Can you work these out from the model? Positions are in its coordinate system, mm. A direction names the side the tool comes from. Coordinates: 2 decimals unless noted, no trailing zeros. Order: outer loops, then holes, each group sorted by start corner. A loop starts at its lowest first (then second) coordinate and runs counter-clockwise, first axis right, second up.
```python
from build123d import *

# Parameters (mm, degrees)
SKETCH_1_W          = 50
SKETCH_1_H          = 50
SKETCH_1_R          = 1.6
EXTRUDE_1_DEPTH     = 20
SKETCH_2_W          = 45
SKETCH_2_H          = 26
CUT_EXTRUDE_1_DEPTH = 16.5
SKETCH_4_R          = 4.6
CUT_EXTRUDE_2_DEPTH = 15
SKETCH_5_R          = 5.15
CUT_EXTRUDE_3_DEPTH = 0.6
CHAMFER_1_SIZE      = 5
SKETCH_6_R          = 3.75
CUT_EXTRUDE_4_DEPTH = 3.3
SKETCH_7_R          = 15
CUT_EXTRUDE_5_DEPTH = 16.5
FILLET_1_R          = 10


with BuildPart() as part:
    # 草图1 → 凸台-拉伸1 (new body)
    with BuildSketch(Plane(origin=(0, 0, 0), x_dir=(1, 0, 0), z_dir=(0, 1, 0))):
        with Locations((25, 25)):
            Rectangle(SKETCH_1_W, SKETCH_1_H)
        with Locations((13.65, 40.5)):
            Circle(SKETCH_1_R, mode=Mode.SUBTRACT)
        with Locations((44.65, 40.5)):
            Circle(SKETCH_1_R, mode=Mode.SUBTRACT)
        with Locations((44.65, 9.5)):
            Circle(SKETCH_1_R, mode=Mode.SUBTRACT)
        with Locations((13.65, 9.5)):
            Circle(SKETCH_1_R, mode=Mode.SUBTRACT)
    extrude(amount=EXTRUDE_1_DEPTH)

    # 草图2 → 切除-拉伸1 (cut)
    with BuildSketch(Plane.XZ):
        with Locations((27.5, -25)):
            Rectangle(SKETCH_2_W, SKETCH_2_H)
    extrude(amount=-CUT_EXTRUDE_1_DEPTH, mode=Mode.SUBTRACT)

    # 草图4 → 切除-拉伸2 (cut)
    with BuildSketch(Plane(origin=(0, 20, 0), x_dir=(1, 0, 0), z_dir=(0, 1, 0))):
        with Locations((29.15, 25)):
            Circle(SKETCH_4_R)
    extrude(amount=-CUT_EXTRUDE_2_DEPTH, mode=Mode.SUBTRACT)

    # 草图5 → 切除-拉伸3 (cut)
    with BuildSketch(Plane.XZ.offset(-16.5)):
        with Locations((29.15, -25)):
            Circle(SKETCH_5_R)
    extrude(amount=-CUT_EXTRUDE_3_DEPTH, mode=Mode.SUBTRACT)

    # 倒角1
    chamfer_1_edges = [part.edges().sort_by_distance(p)[0] for p in [
        (25, 20, -50),
        (50, 8.25, -12),
        (50, 8.25, -38),
        (0, 20, -25),
        (0, 10, -50),
        (50, 10, -50),
        (50, 10, 0),
        (0, 10, 0),
        (25, 20, 0),
    ]]
    chamfer(chamfer_1_edges, length=CHAMFER_1_SIZE)

    # 草图6 → 切除-拉伸4 (cut)
    with BuildSketch(Plane(origin=(0, 20, 0), x_dir=(1, 0, 0), z_dir=(0, 1, 0))):
        with Locations((13.65, 40.5)):
            Circle(SKETCH_6_R)
        with Locations((44.65, 40.5)):
            Circle(SKETCH_6_R)
        with Locations((44.65, 9.5)):
            Circle(SKETCH_6_R)
        with Locations((13.65, 9.5)):
            Circle(SKETCH_6_R)
    extrude(amount=-CUT_EXTRUDE_4_DEPTH, mode=Mode.SUBTRACT)

    # 草图7 → 切除-拉伸5 (cut)
    with BuildSketch(Plane.XZ):
        with Locations((29.15, -25)):
            Circle(SKETCH_7_R)
    extrude(amount=-CUT_EXTRUDE_5_DEPTH, mode=Mode.SUBTRACT)

    # 圆角1
    fillet_1_edges = [part.edges().sort_by_distance(p)[0] for p in [
        (21.666685226, 8.25, -12),
        (36.633314774, 8.25, -12),
        (36.633314774, 8.25, -38),
        (21.666685226, 8.25, -38),
    ]]
    fillet(fillet_1_edges, radius=FILLET_1_R)


solid = part.part
```
1. Please list where these lines run through material, in increasing order: probe 1 along Z at (x, y) = (13.65, 8); probe 2 along X at (y, z) = (18.9, -40.5); probe 3 along Z at (x, y) = (13.65, 19.35).
Completed:
probe 1: z = -50 to -42.1, -38.9 to -38, -12 to -11.1, -7.9 to 0
probe 2: x = 3.9 to 9.9, 17.4 to 40.9, 48.4 to 50
probe 3: z = -45.65 to -44.25, -36.75 to -13.25, -5.75 to -4.35
2. On a 3-axis mill with a long thin cutter (end or side, diameter ignored), from which of +Z, -Z, +X, -X, +Y, -Y can I reach the whole of each face in a straight line? I mean faces 1 (the flat face through (45.4, 16.7, -38.9)), 2 (the flat face through (5, 8, -25)), 3 (the cylindrical face through (36.92, 8.134, -11.792)). Say none if no direction works.
Completed:
face 1: +Y
face 2: +X, -Y
face 3: -Y
3. Imagine slicing it at B-B on z = -28. Please give me the cut outline in (x, y), then the cut area to 3 significant figures.
Completed:
outline: (0, 0) - (5, 0) - (5, 16.5) - (24.96, 16.5) - (24.96, 17.1) - (25.66, 17.1) - (25.66, 20) - (5, 20) - (0, 15) - close; (32.64, 17.1) - (33.34, 17.1) - (33.34, 16.5) - (50, 16.5) - (50, 20) - (32.64, 20) - close
area: 220 mm2
4. Imagine slicing it at A-A on x = 13.65. Please give me the cut outline in (y, z).
Completed:
outline: (0, -50) - (15, -50) - (20, -45) - (20, -44.25) - (16.7, -44.25) - (16.7, -42.1) - (0, -42.1) - close; (0, -38.9) - (16.7, -38.9) - (16.7, -36.75) - (20, -36.75) - (20, -13.25) - (16.7, -13.25) - (16.7, -11.1) - (0, -11.1) - (0, -12) - (16.5, -12) - (16.5, -38) - (0, -38) - close; (0, -7.9) - (16.7, -7.9) - (16.7, -5.75) - (20, -5.75) - (20, -5) - (15, 0) - (0, 0) - close
5. Imagine slicing it at D-D on y = 12.75. Please give me the cut outline in (x, z).
Completed:
outline: (0, -45) - (5, -50) - (45, -50) - (50, -45) - (50, -43) - (45, -38) - (38.95, -38) arc R10 ccw to (35.03, -38.8) arc R15 cw to (23.27, -38.8) arc R10 ccw to (19.35, -38) - (5, -38) - (5, -12) - (19.35, -12) arc R10 ccw to (23.27, -11.2) arc R15 cw to (35.03, -11.2) arc R10 ccw to (38.95, -12) - (45, -12) - (50, -7) - (50, -5) - (45, 0) - (5, 0) - (0, -5) - close; hole circle Ø3.2 at (13.65, -40.5); hole circle Ø3.2 at (13.65, -9.5); hole circle Ø3.2 at (44.65, -40.5); hole circle Ø3.2 at (44.65, -9.5)
6. Imagine slicing it at C-C on x = 29.15. Please give me the cut outline in (y, z), then the cut area to 3 significant figures.
Completed:
outline: (0, -50) - (15, -50) - (20, -45) - (20, -29.6) - (17.1, -29.6) - (17.1, -30.15) - (16.5, -30.15) - (16.5, -40) - (0, -40) - close; (0, -10) - (16.5, -10) - (16.5, -19.85) - (17.1, -19.85) - (17.1, -20.4) - (20, -20.4) - (20, -5) - (15, 0) - (0, 0) - close
area: 447 mm2
7. Thinking about a two-plate mould opening in X: for faces 4 (the flat face through (25, 7, 0)), 5 (the flat face through (3, 7, -48)), 6 (the cylindrical face through (29, 8, -40)), which applies, pulls with the +X half, pulls with the -X half, needs draft (parallel to the pull), parting line crosses it, or undercut?
Completed:
face 4: needs draft
face 5: pulls with the -X half
face 6: undercut
8. I'm going to push flat-ended pins straight in: pin 1 (11.5 mm diameter, centred on x = 30, z = -25.5, fed in from -Y); pin 2 (6 mm diameter, centred on x = 13.65, z = -40.5, fed in from +Y); pin 3 (2 mm diameter, centred on y = 3.5, z = -24, fed in from +X). Where does each tip first touch, or does it pass through?
Completed:
pin 1: stops at y = 16.5
pin 2: stops at y = 16.7
pin 3: stops at x = 5
